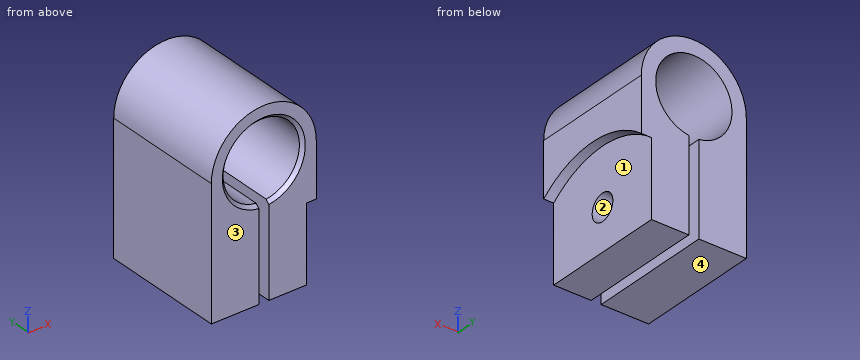
from build123d import *

# Parameters (mm, degrees)
F0_R     = 5.8166
F1_DEPTH = 19.05
F2_SIZE2 = 0.508
F2_SIZE  = 0.508
F4_DEPTH = 25.4
F6_DEPTH = 1.524
F8_D     = 4.0386
F8_DEPTH = 5.715
F8_TIP   = 1.213317848


with BuildPart() as f1:
    # F0 (on Front) → F1 (new body)
    with BuildSketch(Plane.XZ):
        with BuildLine():
            Line((8.001, -19.812), (8.001, 0))
            ThreePointArc((8.001, 0), (0, 8.001), (-8.001, 0))
            Line((-8.001, 0), (-8.001, -19.812))
            Line((-8.001, -19.812), (8.001, -19.812))
        make_face()
        Circle(F0_R, mode=Mode.SUBTRACT)
    extrude(amount=-F1_DEPTH)

    # F2
    f2_edges = [f1.edges().sort_by_distance(p)[0] for p in [
        (-5.8166, 0, 0),
    ]]
    chamfer(f2_edges, length=F2_SIZE, length2=F2_SIZE2)

    # F3 (on face) → F4 (cut)
    with BuildSketch(Plane.XZ):
        with BuildLine():
            Line((-0.762, -6.2785285824), (-0.762, -19.812))
            Line((-0.762, -19.812), (0.762, -19.812))
            Line((0.762, -19.812), (0.762, -6.2785285824))
            ThreePointArc((0.762, -6.2785285824), (0, -6.3246), (-0.762, -6.2785285824))
        make_face()
        with BuildLine():
            Line((-0.762, 0), (-0.762, -6.2785285824))
            ThreePointArc((-0.762, -6.2785285824), (0, -6.3246), (0.762, -6.2785285824))
            Line((0.762, -6.2785285824), (0.762, 0))
            Line((0.762, 0), (-0.762, 0))
        make_face()
    extrude(amount=-F4_DEPTH, mode=Mode.SUBTRACT)

    # F5 (on face) → F6 (cut)
    with BuildSketch(Plane.YZ.offset(8.001)):
        with BuildLine():
            Line((19.05, -19.812), (19.05, -8.2424463785))
            ThreePointArc((19.05, -8.2424463785), (9.525, -4.826), (0, -8.2424463785))
            Line((0, -8.2424463785), (0, -19.812))
            Line((0, -19.812), (19.05, -19.812))
        make_face()
        with BuildLine():
            ThreePointArc((0, -8.2424463785), (3.1281825882, -33.3641556588), (24.511, -19.812))
            ThreePointArc((24.511, -19.812), (23.0771556588, -13.4151825882), (19.05, -8.2424463785))
            Line((19.05, -8.2424463785), (19.05, -19.812))
            Line((19.05, -19.812), (0, -19.812))
            Line((0, -19.812), (0, -8.2424463785))
        make_face()
    extrude(amount=-F6_DEPTH, mode=Mode.SUBTRACT)

    # F8
    with Locations(Plane.YZ.offset(6.477)):
        with Locations((9.525, -13.462)):
            Hole(F8_D / 2, depth=F8_DEPTH)
            with Locations((0, 0, -(F8_DEPTH + F8_TIP / 2))):  # 118° drill point
                Cone(0, F8_D / 2, F8_TIP, mode=Mode.SUBTRACT)


solid = f1.part
Check sheet for the modelled part. Datum: model origin and axes. Units: mm. Face numbers are marked on the shaded views. Round coordinates to 2 decimals unless told otherwise and drop trailing zeros. Loops run counter-clockwise (first coordinate to the right, second up) from the corner with the lowest first, then second, coordinate; pieces in that order, holes last. Notation, with made-up numbers: M 73,31.5 L 118,31.5 A19 ccw 118,35.5 Z; hole C 22.25,87.5 d8. An arc over 180 degrees is marked long. One line per question, with ' | ' between items. Start each with the question number.
Item 1: Scan lines: probe 1 along Z at (x, y) = (2.5, 10.75); probe 2 along X at (y, z) = (11.75, -17.25); probe 3 along X at (y, z) = (18.25, -6.25). Record each from-to range of solid material in increasing order.
Item 2: Release check for a two-part mould opening along Y. For the marked faces 1, 2, 3 and 4 record: released by +Y, released by -Y, zero draft, split by the parting line, or undercut.
Item 3: Section check C-C (y = 5.75). Record the boundary of the cut face in (x, z), and give its area (3 significant figures).
Item 4: Section check B-B (x = 0). Record the boundary of the cut face in (y, z), and give its area (3 significant figures).
Item 5: Section check A-A (y = 8.5). Record the boundary of the cut face in (x, z), and give its area (3 significant figures).
Item 6: Section check D-D (y = 13.75). Record the boundary of the cut face in (x, z), and give its area (3 significant figures).
Item 7: Gauge pin test, flat ends, axial feed: pin 1 Ø7 at (y, z) = (6, -13.5) entering from +X; pin 2 Ø4 at (x, y) = (0.5, 16.5) entering from +Z; pin 3 Ø1 at (y, z) = (5.5, 4.5) entering from +X. Record the tip position at first contact, or that the pin passes through.
Worked out:
1) probe 1: -19.81 to -15.07, -11.86 to -5.25, 5.25 to 7.6 | probe 2: -8 to -0.76, 0.76 to 6.48 | probe 3: -8 to -0.76, 0.76 to 8
2) face 1: undercut | face 2: undercut | face 3: released by -Y | face 4: zero draft
3) outline: M -8,-19.81 L -0.76,-19.81 L -0.76,-5.77 A5.82 cw long 0.76,-5.77 L 0.76,-19.81 L 6.48,-19.81 L 6.48,-5.31 L 8,-5.31 L 8,0 A8 ccw -8,0 Z | area: 268 mm^2
4) outline: M 0,6.32 L 0.51,5.82 L 19.05,5.82 L 19.05,8 L 0,8 Z | area: 41.5 mm^2
5) outline: M -8,-19.81 L -0.76,-19.81 L -0.76,-5.77 A5.82 cw long 0.76,-5.77 L 0.76,-11.72 L 6.48,-11.72 L 6.48,-4.86 L 8,-4.86 L 8,0 A8 ccw -8,0 Z; M 0.76,-19.81 L 6.48,-19.81 L 6.48,-15.2 L 0.76,-15.2 Z | area: 247 mm^2
6) outline: M -8,-19.81 L -0.76,-19.81 L -0.76,-5.77 A5.82 cw long 0.76,-5.77 L 0.76,-19.81 L 6.48,-19.81 L 6.48,-5.43 L 8,-5.43 L 8,0 A8 ccw -8,0 Z | area: 268 mm^2
7) pin 1: x = 6.48 | pin 2: z = 8 | pin 3: x = 6.93
